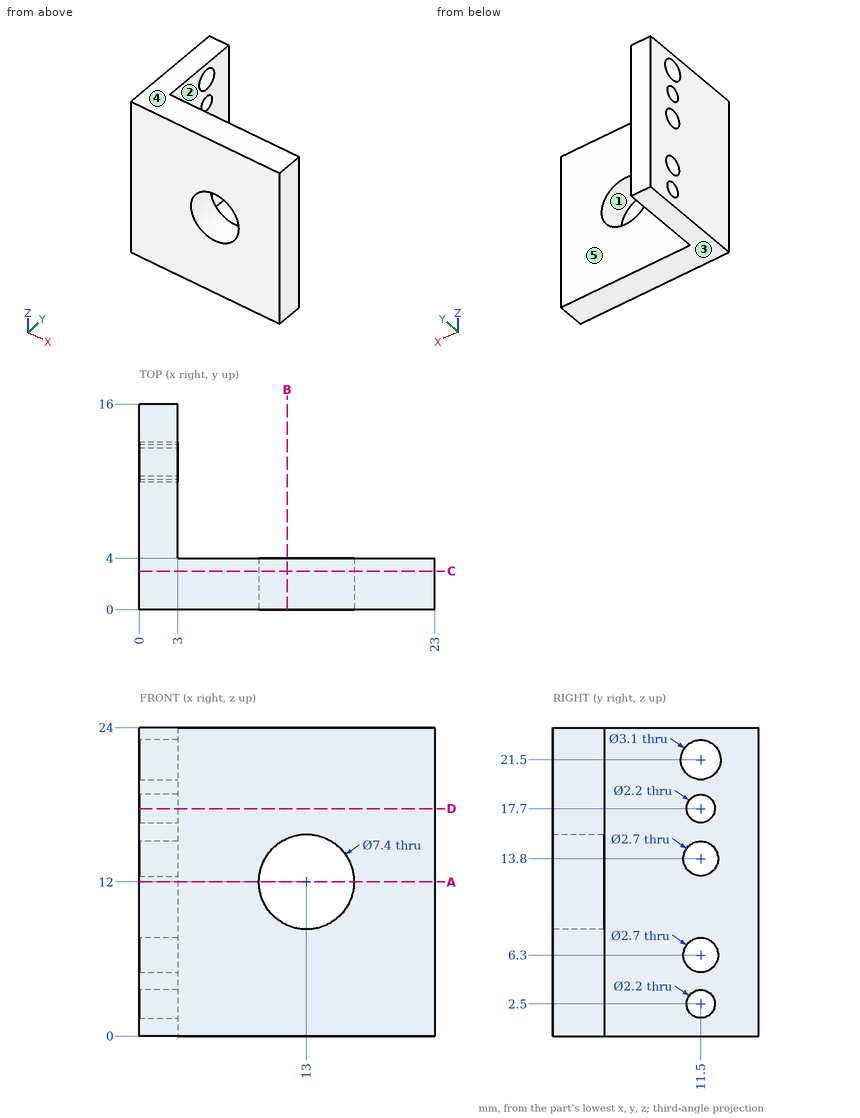
Here's the drawing with two shaded views (mm, measured from the low corner). I have some questions. A direction names the side the tool comes from. Coordinates: 2 decimals unless noted, no trailing zeros. Loops run counter-clockwise (first coordinate to the right, second up) from the corner with the lowest first, then second, coordinate; pieces in that order, holes last. Notation, with made-up numbers: M 66,-7 L 100,-7 A21 cw 100,-3 Z; hole C -40,42.5 d8. An arc over 180 degrees is marked long. Put each result on its own line as item: value. Start each with the question number.
(1) Imagine slicing it at C-C on y = 3. List the corners of the cut face in (x, z) for me, and give its area (3 significant figures).
(2) Which directions (+Z, -Z, +X, -X, +Y, -Y) give clear straight access to the entire face, cutting with the end or side of a thin tool? Please do the marked faces 4 and 5.
(3) We'd pull the mould along Z, two halves only. Please class the marked faces 1, 2 and 3: +Z half, -Z half, draft (parallel to the pull), parting line (faces both ways), or undercut.
(4) Imagine slicing it at D-D on z = 17.7. List the corners of the cut face in (x, y) for me, and give its area (3 significant figures).
(5) Imagine slicing it at A-A on z = 12. List the corners of the cut face in (x, y) for me, and give its area (3 significant figures).
(6) I need wall thicknesses on probe 1 along Y at (x, z) = (0.8, 21.5); probe 2 along Y at (x, z) = (2.2, 2.5); probe 3 along X at (y, z) = (11.5, 10.75). Which ranges of each line are inside material? Lowest first, please.
(7) Imagine slicing it at B-B on x = 11.5. List the corners of the cut face in (y, z) for me.
(8) Will these pins go through, and if not, where does the flat tip stop? pin 1 Ø4.5 at (y, z) = (11.5, 6.3) entering from +X; pin 2 Ø8.5 at (x, z) = (13, 12) entering from -Y; pin 3 Ø8 at (x, z) = (10.5, 10.5) entering from +Y.
Worked answers:
1. outline: M 0,0 L 23,0 L 23,24 L 0,24 Z; hole C 13,12 d7.4
1. area: 509 mm2
2. face 4: +Z, +X, -X, +Y, -Y
2. face 5: +Z, -Z, +X, +Y
3. face 1: undercut
3. face 2: draft
3. face 3: -Z half
4. outline: M 0,0 L 23,0 L 23,4 L 3,4 L 3,10.4 L 0,10.4 Z; M 0,12.6 L 3,12.6 L 3,16 L 0,16 Z
4. area: 121 mm2
5. outline: M 0,0 L 9.3,0 L 9.3,4 L 3,4 L 3,16 L 0,16 Z; M 16.7,0 L 23,0 L 23,4 L 16.7,4 Z
5. area: 98.4 mm2
6. probe 1: y = 0 to 9.95, 13.05 to 16
6. probe 2: y = 0 to 10.4, 12.6 to 16
6. probe 3: x = 0 to 3
7. outline: M 0,0 L 4,0 L 4,8.62 L 0,8.62 Z; M 0,15.38 L 4,15.38 L 4,24 L 0,24 Z
8. pin 1: stops at x = 3
8. pin 2: stops at y = 0
8. pin 3: stops at y = 4
